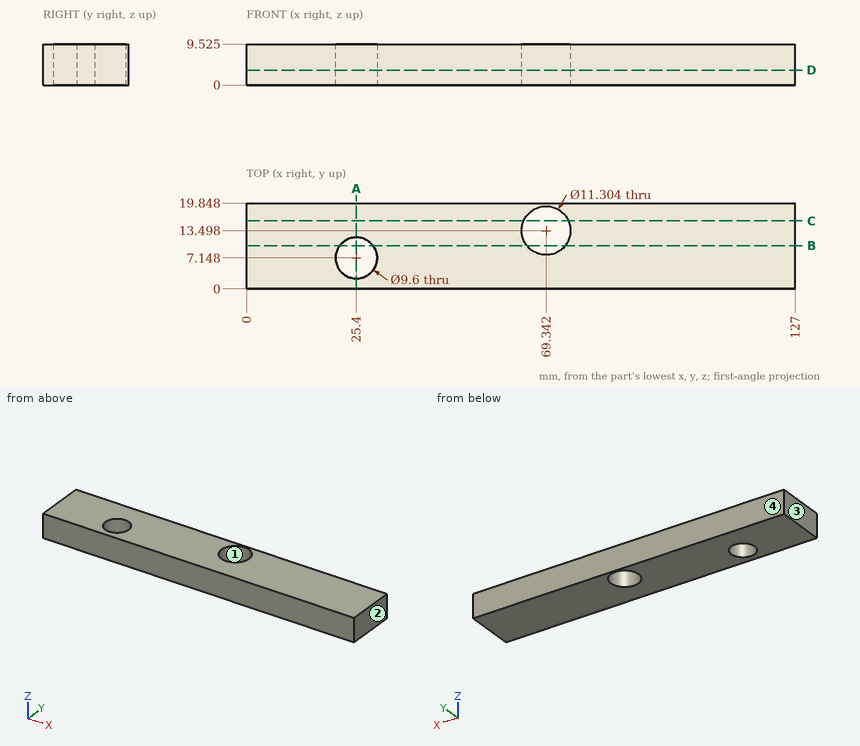
Could you check a few things on this drawing? It's one solid part, dimensions in mm from its lowest x, y, z. Round coordinates to 2 decimals unless told otherwise and drop trailing zeros. Loops run counter-clockwise (first coordinate to the right, second up) from the corner with the lowest first, then second, coordinate; pieces in that order, holes last. Notation, with made-up numbers: M 56.25,75.5 L 113.25,75.5 A36 cw 113.25,112.5 Z; hole C -17,56.25 d9. An arc over 180 degrees is marked long. Write item = value, one per line. Start each with the question number.
(1) Suppose I cut it at D-D on z = 3.5. Write out the boundary of the cut face in (x, y) (1 decimal).
(2) Suppose I cut it at B-B on y = 10. Write out the boundary of the cut face in (x, z) (1 decimal).
(3) I need wall thicknesses on line 1 along Y through (x, z) = (25.4, 6.5); line 2 along X through (y, z) = (13.25, 3.25) (1 decimal); line 3 along X through (y, z) = (16.75, 7) (1 decimal). Which ranges of each line are inside material? Lowest first, please.
(4) Suppose I cut it at C-C on y = 15.75. Write out the boundary of the cut face in (x, z) (1 decimal), plus the area to 3 significant figures.
(5) If we mould it in two halves opening along X, with no side actions, what happens to the marked faces 1, 2, 3 and 4? For each: released by +X, released by -X, zero draft, split by the parting line, or undercut.
(6) Suppose I cut it at A-A on x = 25.4. Write out the boundary of the cut face in (y, z) (1 decimal).
Answer block:
q1.outline = M 0,0 L 127,0 L 127,19.8 L 0,19.8 Z; hole C 25.4,7.1 d9.6; hole C 69.3,13.5 d11.3
q2.outline = M 0,0 L 21.5,0 L 21.5,9.5 L 0,9.5 Z; M 29.3,0 L 64.9,0 L 64.9,9.5 L 29.3,9.5 Z; M 73.8,0 L 127,0 L 127,9.5 L 73.8,9.5 Z
q3.line_1 = 0 to 2.35, 11.95 to 19.85
q3.line_2 = 0 to 63.7, 75 to 127
q3.line_3 = 0 to 64.7, 74 to 127
q4.outline = M 0,0 L 64.2,0 L 64.2,9.5 L 0,9.5 Z; M 74.5,0 L 127,0 L 127,9.5 L 74.5,9.5 Z
q4.area = 1,110 mm²
q5.face_1 = undercut
q5.face_2 = released by +X
q5.face_3 = released by -X
q5.face_4 = zero draft
q6.outline = M 0,0 L 2.3,0 L 2.3,9.5 L 0,9.5 Z; M 11.9,0 L 19.8,0 L 19.8,9.5 L 11.9,9.5 Z
